Verification items for the finished model (mm, model axes). Face numbers are marked on the shaded views. A direction names the side the tool comes from. Give positions to 0.01 mm unless a question says otherwise; leave off trailing zeros. Order: outer loops, then holes, each group sorted by start corner. A loop starts at its lowest first (then second) coordinate and runs counter-clockwise, first axis right, second up. Notation, with made-up numbers: M -7.5,-2.5 L -2.5,-2.5 A28 cw -2.5,21.5 Z; hole C -37.5,15 d5. An arc over 180 degrees is marked long. Answer as a JSON object with one key per item and string values.
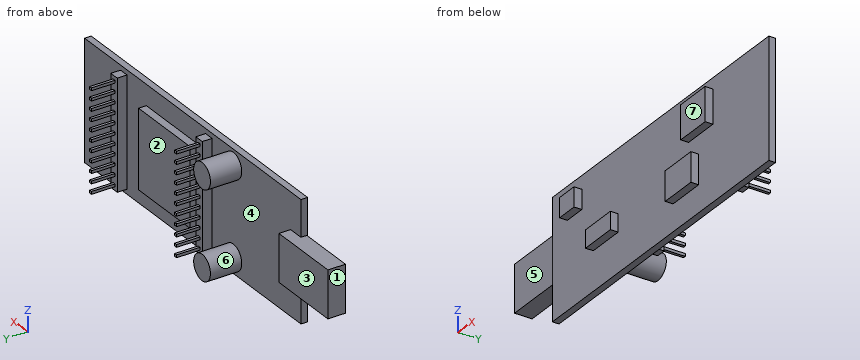
```python
from build123d import *

# Parameters (mm, degrees)
SKETCH1_W                = 84
SKETCH1_H                = 30.5
BOSS_EXTRUDE1_DEPTH      = 1.7
BOSS_EXTRUDE2_DEPTH      = 3
BOSS_EXTRUDE2_DEPTH_BACK = 1.5
SKETCH2_W                = 19
SKETCH2_H                = 12
SKETCH3_W                = 20
SKETCH3_H                = 20
BOSS_EXTRUDE3_DEPTH      = 2
SKETCH4_W                = 5.627780268
SKETCH4_H                = 4.971205903
SKETCH4_W_2              = 9.661022794
SKETCH4_H_2              = 4.502224215
SKETCH4_W_3              = 9.473430118
SKETCH4_H_3              = 8.629263078
SKETCH4_W_4              = 9.942411808
SKETCH4_H_4              = 7.503707025
BOSS_EXTRUDE4_DEPTH      = 2
SKETCH5_R                = 3.25
BOSS_EXTRUDE5_DEPTH      = 8
SKETCH6_W                = 2.5
SKETCH6_H                = 28
BOSS_EXTRUDE6_DEPTH      = 2.5
SKETCH7_W                = 0.7
SKETCH7_H                = 0.7
BOSS_EXTRUDE7_DEPTH      = 6


with BuildPart() as part:
    # Sketch1 → Boss-Extrude1 (new body)
    with BuildSketch(Plane(origin=(0, 0, 0), x_dir=(1, 0, 0), z_dir=(0, 1, 0))):
        Rectangle(SKETCH1_W, SKETCH1_H)
    extrude(amount=BOSS_EXTRUDE1_DEPTH)

    # Sketch2 → Boss-Extrude2 (add, two sides: drawn at the far end of the back side and taken through both)
    with BuildSketch(Plane(origin=(0, 1.7, 0), x_dir=(1, 0, 0), z_dir=(0, 1, 0)).offset(-BOSS_EXTRUDE2_DEPTH_BACK)):
        with Locations((-47.5, 0)):
            Rectangle(SKETCH2_W, SKETCH2_H)
    extrude(amount=BOSS_EXTRUDE2_DEPTH + BOSS_EXTRUDE2_DEPTH_BACK)

    # Sketch3 → Boss-Extrude3 (add)
    with BuildSketch(Plane(origin=(0, 1.7, 0), x_dir=(1, 0, 0), z_dir=(0, 1, 0))):
        with Locations((8, 0)):
            Rectangle(SKETCH3_W, SKETCH3_H)
    extrude(amount=BOSS_EXTRUDE3_DEPTH)

    # Sketch4 → Boss-Extrude4 (add)
    with BuildSketch(Plane.XZ):
        with Locations((-33.387789234, 9.379633781)):
            Rectangle(SKETCH4_W, SKETCH4_H)
        with Locations((-21.288061657, -3.048380979)):
            Rectangle(SKETCH4_W_2, SKETCH4_H_2)
        with Locations((15.5738991, 8.160281389)):
            Rectangle(SKETCH4_W_3, SKETCH4_H_3)
        with Locations((9.805424325, -4.642918722)):
            Rectangle(SKETCH4_W_4, SKETCH4_H_4)
    extrude(amount=BOSS_EXTRUDE4_DEPTH)

    # Sketch5 → Boss-Extrude5 (add)
    with BuildSketch(Plane(origin=(0, 1.7, 0), x_dir=(1, 0, 0), z_dir=(0, 1, 0))):
        with Locations(Location((-15.754077727, 11.25, 0), (0, 0, 270))):
            Circle(SKETCH5_R)
        with Locations(Location((-15.754077727, -11.25, 0), (0, 0, 90))):
            Circle(SKETCH5_R)
    extrude(amount=BOSS_EXTRUDE5_DEPTH)

    # Sketch6 → Boss-Extrude6 (add)
    with BuildSketch(Plane(origin=(0, 1.7, 0), x_dir=(1, 0, 0), z_dir=(0, 1, 0))):
        with Locations((-6.25, 0)):
            Rectangle(SKETCH6_W, SKETCH6_H)
        with Locations((26.75, 0)):
            Rectangle(SKETCH6_W, SKETCH6_H)
    extrude(amount=BOSS_EXTRUDE6_DEPTH)

    # Sketch7 → Boss-Extrude7 (add)
    with BuildSketch(Plane(origin=(0, 4.2, 0), x_dir=(1, 0, 0), z_dir=(0, 1, 0))):
        with Locations((-6.25, 2.54)):
            Rectangle(SKETCH7_W, SKETCH7_H)
        with Locations((-6.25, 0)):
            Rectangle(SKETCH7_W, SKETCH7_H)
        with Locations((-6.25, 5.08)):
            Rectangle(SKETCH7_W, SKETCH7_H)
        with Locations((-6.25, 7.62)):
            Rectangle(SKETCH7_W, SKETCH7_H)
        with Locations((-6.25, 10.16)):
            Rectangle(SKETCH7_W, SKETCH7_H)
        with Locations((-6.25, 12.7)):
            Rectangle(SKETCH7_W, SKETCH7_H)
        with Locations((-6.25, -2.54)):
            Rectangle(SKETCH7_W, SKETCH7_H)
        with Locations((-6.25, -5.08)):
            Rectangle(SKETCH7_W, SKETCH7_H)
        with Locations((-6.25, -7.62)):
            Rectangle(SKETCH7_W, SKETCH7_H)
        with Locations((-6.25, -10.16)):
            Rectangle(SKETCH7_W, SKETCH7_H)
        with Locations((-6.25, -12.7)):
            Rectangle(SKETCH7_W, SKETCH7_H)
        with Locations((26.75, 2.54)):
            Rectangle(SKETCH7_W, SKETCH7_H)
        with Locations((26.75, 10.16)):
            Rectangle(SKETCH7_W, SKETCH7_H)
        with Locations((26.75, -12.7)):
            Rectangle(SKETCH7_W, SKETCH7_H)
        with Locations((26.75, -2.54)):
            Rectangle(SKETCH7_W, SKETCH7_H)
        with Locations((26.75, 7.62)):
            Rectangle(SKETCH7_W, SKETCH7_H)
        with Locations((26.75, 12.7)):
            Rectangle(SKETCH7_W, SKETCH7_H)
        with Locations((26.75, 0)):
            Rectangle(SKETCH7_W, SKETCH7_H)
        with Locations((26.75, -5.08)):
            Rectangle(SKETCH7_W, SKETCH7_H)
        with Locations((26.75, -10.16)):
            Rectangle(SKETCH7_W, SKETCH7_H)
        with Locations((26.75, -7.62)):
            Rectangle(SKETCH7_W, SKETCH7_H)
        with Locations((26.75, 5.08)):
            Rectangle(SKETCH7_W, SKETCH7_H)
    extrude(amount=BOSS_EXTRUDE7_DEPTH)


solid = part.part
```
Q1. Release check for a two-part mould opening along X. For the marked faces 1, 2, 3 and 4 record: +X half, -X half, draft (parallel to the pull), parting line (faces both ways), or undercut.
Resolved:
{"face 1": "-X half", "face 2": "undercut", "face 3": "draft", "face 4": "undercut"}
Q2. Gauge pin test, flat ends, axial feed: pin 1 Ø0.6 at (x, y) = (26.5, 6.5) entering from -Z; pin 2 Ø0.8 at (y, z) = (6.5, 10) entering from +X; pin 3 Ø5 at (y, z) = (6.5, 12) entering from +X; pin 4 Ø1 at (x, y) = (24.5, 7.5) entering from -Z. Record the tip position at first contact, or that the pin passes through.
Resolved:
{"pin 1": "stops at z = -13.05", "pin 2": "stops at x = 27.1", "pin 3": "stops at x = 28", "pin 4": "passes through"}
Q3. Material ranges on L1, parallel to X at y = 9, z = 2.5; L2, parallel to Y at x = -23.5, z = -3; L3, parallel to X at y = 5.5, z = 11, recorded low to high.
Resolved:
{"L1": "x = -6.6 to -5.9, 26.4 to 27.1", "L2": "y = -2 to 1.7", "L3": "x = -18.99 to -12.51"}
Q4. Tool access check on the marked faces 5, 6 and 7. Record the directions out of +Z, -Z, +X, -X, +Y, -Y that give a thin tool (end or side, any length) a straight path to the whole face; none if there is none.
Resolved:
{"face 5": "+Z, -Z, -X, -Y", "face 6": "+Y", "face 7": "+Z, -Z, +X, -X, -Y"}
Q5. Section check A-A on x = 7.5. Record the cut outline in (y, z).
Resolved:
{"outline": "M -2,-8.39 L 0,-8.39 L 0,-15.25 L 1.7,-15.25 L 1.7,-10 L 3.7,-10 L 3.7,10 L 1.7,10 L 1.7,15.25 L 0,15.25 L 0,-0.89 L -2,-0.89 Z"}
